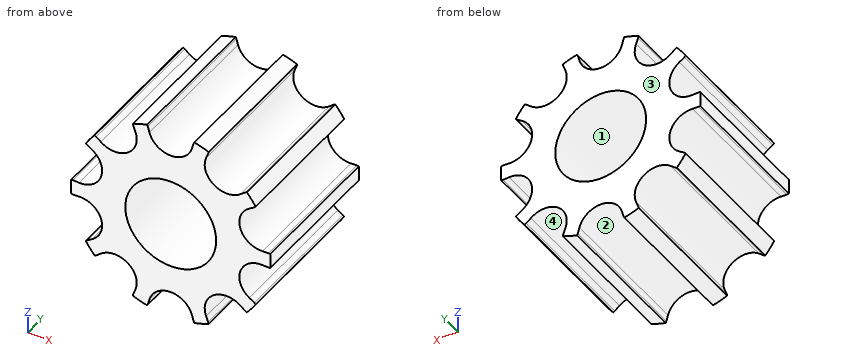
from build123d import *

# Parameters (mm, degrees)
SKETCH1_R          = 4.393648446
TOOTHOD_DEPTH      = 3.4925
TOOTHPROFILE_DEPTH = 4.4925
TOOTHPATTERN_COUNT = 10
SKETCH7_R          = 2
BORE_DEPTH         = 5.5085
BORE_DEPTH_BACK    = 5.5085
CUT_EXTRUDE1_START = 3.175
SKETCH11_R         = 5.536648446
CUT_EXTRUDE1_DEPTH = 2.3335
CUT_EXTRUDE2_START = -3.175
SKETCH11_2_R       = 5.536648446
CUT_EXTRUDE2_DEPTH = 2.3335


with BuildPart() as part:
    # Sketch1 → ToothOD (new body, symmetric)
    with BuildSketch(Plane(origin=(0, 0, 0), x_dir=(1, 0, 0), z_dir=(0, 1, 0))):
        Circle(SKETCH1_R)
    extrude(amount=TOOTHOD_DEPTH, both=True)

    # Sketch2 → ToothProfile (cut, symmetric)
    with BuildSketch(Plane(origin=(0, 0, 0), x_dir=(1, 0, 0), z_dir=(0, 1, 0))):
        with BuildLine():
            ThreePointArc((-0.937033068, 3.943710441), (-0.590385173, 3.425535831), (0, 3.225248446))
            ThreePointArc((0, 3.225248446), (0.590385173, 3.425535831), (0.937033068, 3.943710441))
            ThreePointArc((0.937033068, 3.943710441), (0.971699064, 4.069821903), (1.007805813, 4.195528446))
            ThreePointArc((1.007805813, 4.195528446), (1.021661234, 4.233200647), (1.040426249, 4.268683624))
            ThreePointArc((1.040426249, 4.268683624), (0, 4.393648446), (-1.040426249, 4.268683624))
            ThreePointArc((-1.040426249, 4.268683624), (-1.021661234, 4.233200647), (-1.007805813, 4.195528446))
            ThreePointArc((-1.007805813, 4.195528446), (-0.971699064, 4.069821903), (-0.937033068, 3.943710441))
        make_face()
    toothprofile = extrude(amount=TOOTHPROFILE_DEPTH, both=True, mode=Mode.SUBTRACT)

    # ToothPattern: ToothProfile ×10 about axis
    toothpattern_axis = Axis((0, 0, 0), (0, 1, 0))
    for i in range(1, TOOTHPATTERN_COUNT):
        add(toothprofile.rotate(toothpattern_axis, i * 360 / TOOTHPATTERN_COUNT), mode=Mode.SUBTRACT)

    # Sketch4 → Flange (revolve)
    with BuildSketch(Plane.XY):
        with BuildLine():
            Line((0, -3.4925), (4.647648446, -3.4925))
            ThreePointArc((4.647648446, -3.4925), (4.839929254, -3.531494589), (5.028648446, -3.585137424))
            ThreePointArc((5.028648446, -3.585137424), (5.304690043, -3.90309066), (5.536648446, -4.2545))
            Line((5.536648446, -4.2545), (5.536648446, -4.5085))
            Line((5.536648446, -4.5085), (0, -4.5085))
            Line((0, -4.5085), (0, -3.4925))
        make_face()
        with BuildLine():
            Line((5.536648446, 4.5085), (5.536648446, 4.2545))
            ThreePointArc((5.536648446, 4.2545), (5.304690043, 3.90309066), (5.028648446, 3.585137424))
            ThreePointArc((5.028648446, 3.585137424), (4.839929254, 3.531494589), (4.647648446, 3.4925))
            Line((4.647648446, 3.4925), (0, 3.4925))
            Line((0, 3.4925), (0, 4.5085))
            Line((0, 4.5085), (5.536648446, 4.5085))
        make_face()
    revolve(axis=Axis((0, 8.73125, 0), (0, -1, 0)))

    # Sketch7 → Bore (cut, two sides)
    with BuildSketch(Plane.XZ) as bore_sk:
        Circle(SKETCH7_R)
    extrude(amount=BORE_DEPTH, mode=Mode.SUBTRACT)
    extrude(bore_sk.sketch, amount=-BORE_DEPTH_BACK, mode=Mode.SUBTRACT)

    # Sketch11 → Cut-Extrude1 (cut, through all)
    with BuildSketch(Plane(origin=(0, 0, 0), x_dir=(1, 0, 0), z_dir=(0, 1, 0)).offset(CUT_EXTRUDE1_START)):
        Circle(SKETCH11_R)
    extrude(amount=CUT_EXTRUDE1_DEPTH, mode=Mode.SUBTRACT)

    # Sketch11_2 → Cut-Extrude2 (cut, through all)
    with BuildSketch(Plane(origin=(0, 0, 0), x_dir=(1, 0, 0), z_dir=(0, 1, 0)).offset(CUT_EXTRUDE2_START)):
        Circle(SKETCH11_2_R)
    extrude(amount=-CUT_EXTRUDE2_DEPTH, mode=Mode.SUBTRACT)


solid = part.part
Model file for the job. Use its own axes, mm. Face numbers are marked on the shaded views. Round coordinates to 2 decimals unless told otherwise and drop trailing zeros. Loops run counter-clockwise (first coordinate to the right, second up) from the corner with the lowest first, then second, coordinate; pieces in that order, holes last. Notation, with made-up numbers: (56, -9.5) - (99, -9.5) arc R15 cw to (99, 18.5) - close; hole circle Ø7 at (34, 45). An arc over 180 degrees is marked (long way). Write each question's results on one line, items separated by ' | '.
(1) Saw through at A-A, the plane x = 0. List the corners of the cut face in (y, z) (3 decimals).
Answer below:
outline: (-3.175, -3.225) - (3.175, -3.225) - (3.175, -2) - (-3.175, -2) - close; (-3.175, 2) - (3.175, 2) - (3.175, 3.225) - (-3.175, 3.225) - close
(2) Pin check, flat tips, straight feed: pin 1 (3 mm diameter, centred on x = 0.5, z = 0.5, fed in from -Y) (3 decimals); pin 2 (3 mm diameter, centred on y = -1.5, z = 3, fed in from +X); pin 3 (3 mm diameter, centred on x = 0, z = 0, fed in from +Y). Stop position of each tip, or through.
Answer below:
pin 1: stops at y = -3.175 | pin 2: stops at x = 3.74 | pin 3: passes through
(3) Wall check: L1, parallel to X at y = 1.75, z = 2.75; L2, parallel to X at y = -2.5, z = 1.25; L3, parallel to X at y = -2.25, z = 1. Give the ranges that are in metal, low to high.
Answer below:
L1: x = -3.43 to -3.21, -1.74 to 1.74, 3.21 to 3.43 | L2: x = -3.02 to -1.56, 1.56 to 3.02 | L3: x = -3.07 to -1.73, 1.73 to 3.07
(4) Saw through at B-B, the plane z = 0. List the corners of the cut face in (x, y) (3 decimals), then the cut area to 3 significant figures.
Answer below:
outline: (-4.394, -3.175) - (-2, -3.175) - (-2, 3.175) - (-4.394, 3.175) - close; (2, -3.175) - (4.394, -3.175) - (4.394, 3.175) - (2, 3.175) - close | area: 30.4 mm^2
(5) Mould opens along Z. For the marked faces 1, 2, 3 and 4 say: released by +Z, released by -Z, zero draft, split by the parting line, or undercut.
Answer below:
face 1: undercut | face 2: released by -Z | face 3: zero draft | face 4: undercut
